from build123d import *

# Parameters (mm, degrees)
SKETCH_R    = 5.15
SKETCH_R_2  = 4.15
PAD_DEPTH   = 9
FILLET_R    = 0.2
FILLET001_R = 0.2


with BuildPart() as part:
    # Sketch → Pad (new body)
    with BuildSketch(Plane.XY):
        Circle(SKETCH_R)
        Circle(SKETCH_R_2, mode=Mode.SUBTRACT)
    extrude(amount=PAD_DEPTH)

    # Fillet
    fillet_edges = [part.edges().sort_by_distance(p)[0] for p in [
        (-5.15, 0, 9),
        (-4.15, 0, 9),
    ]]
    fillet(fillet_edges, radius=FILLET_R)

    # Fillet001
    fillet001_edges = [part.edges().sort_by_distance(p)[0] for p in [
        (-5.15, 0, 0),
        (-4.15, 0, 0),
    ]]
    fillet(fillet001_edges, radius=FILLET001_R)


solid = part.part
The listing builds one solid part. Answer for the finished solid, in the listing's coordinates (mm). Coordinates: 2 decimals unless noted, no trailing zeros. Write each loop counter-clockwise with the first axis right and the second up, starting at its lowest first coordinate (ties: lowest second). Pieces come first, ordered by that corner, then holes. Notation, with made-up numbers: (-18, 8.25) - (-11, 8.25) arc R37 cw to (-11, 44.25) - close; hole circle Ø10 at (-20, -2). An arc over 180 degrees is marked (long way). Put each result on its own line as item: value.
1. Determine the mould class of faces 1 (the face through (4.91, 1.55, 4.44)), 2 (the face through (-0.9, -4.05, 4.44)) for opening direction Y: pulls with the +Y half, pulls with the -Y half, needs draft (parallel to the pull), parting line crosses it, or undercut.
Answer sheet:
face 1: parting line crosses it
face 2: undercut
2. Flat-ended cylindrical pins translate along their axes: pin 1 Ø4 at (y, z) = (-3.5, 6.5) entering from -X; pin 2 Ø3 at (x, z) = (-3.5, 2) entering from +Y; pin 3 Ø4 at (x, z) = (-3, 5.5) entering from -Y; pin 4 Ø3 at (y, z) = (-1.5, 1.5) entering from +X. Find the tip coordinate at first contact, or state that the pin passes through.
Answer sheet:
pin 1: stops at x = -4.93
pin 2: stops at y = 4.75
pin 3: stops at y = -5.05
pin 4: stops at x = 5.15
3. Find the intervals of material crossed by line 1 along Y through (x, z) = (0, 3); line 2 along X through (y, z) = (2.75, 3.75); line 3 along X through (y, z) = (1.25, 4), in increasing order. Write a range as from..to.
Answer sheet:
line 1: y = -5.15..-4.15, 4.15..5.15
line 2: x = -4.35..-3.11, 3.11..4.35
line 3: x = -5..-3.96, 3.96..5
4. The part is cut by section C-C on z = 5.75. Give the vertices of the cut face in (x, y), plus the area to 3 significant figures.
Answer sheet:
outline: circle Ø10.3 at (0, 0); hole circle Ø8.3 at (0, 0)
area: 29.2 mm^2
5. The part is cut by section A-A on x = 0. Give the vertices of the cut face in (y, z).
Answer sheet:
outline: (-5.15, 0.2) arc R0.2 ccw to (-4.95, 0) - (-4.35, 0) arc R0.2 ccw to (-4.15, 0.2) - (-4.15, 8.8) arc R0.2 ccw to (-4.35, 9) - (-4.95, 9) arc R0.2 ccw to (-5.15, 8.8) - close; (4.15, 0.2) arc R0.2 ccw to (4.35, 0) - (4.95, 0) arc R0.2 ccw to (5.15, 0.2) - (5.15, 8.8) arc R0.2 ccw to (4.95, 9) - (4.35, 9) arc R0.2 ccw to (4.15, 8.8) - close
